Part model, mm, in its own coordinate system. A direction names the side the tool comes from. Coordinates: 2 decimals unless noted, no trailing zeros. Write each loop counter-clockwise with the first axis right and the second up, starting at its lowest first coordinate (ties: lowest second). Pieces come first, ordered by that corner, then holes. Notation, with made-up numbers: M 13,19.5 L 31,19.5 A22 ccw 31,30.5 Z; hole C 29,70.5 d3. An arc over 180 degrees is marked long. Use a Markdown table: item, result. Add a question column.
Q1. Slice it at B-B on y = 60.5. Write the cut outline in (x, z).
Q2. Tool access for faces 4 (the flat face through (-27.1, 42, 0)), 5 (the flat face through (25, 33, 0)), 6 (the flat face through (28, 57, -5)), 7 (the cylindrical face through (-28.53, 42.536, 7.325)), 8 (the flat face through (-28, 31, -15)): list every direction of +Z, -Z, +X, -X, +Y, -Y with a clear straight run to the whole face (end or side of a thin tool).
Q3. Pin check, flat tips, straight feed: pin 1 Ø1 at (x, z) = (5, -26) entering from -Y; pin 2 Ø5 at (x, z) = (9.5, 37.5) entering from -Y; pin 3 Ø5.5 at (x, y) = (28, 53) entering from -Z; pin 4 Ø4 at (x, z) = (-8.49, 8.49) entering from +Y. Stop position of each tip, or through.
Q4. Wall check: L1, parallel to Y at x = -27.5, z = -0.5; L2, parallel to X at y = 1.25, z = 0; L3, parallel to X at y = 30.5, z = 11. Give the ranges that are in metal, low to high. Write a range as from..to.
Q5. Mould opens along X. For faces 1 (the cylindrical face through (-24, 6, 0)), 2 (the cylindrical face through (-27, 5, -17)), 3 (the cylindrical face through (-32, 5, 0)) say: released by +X, released by -X, zero draft, split by the parting line, or undercut.
Q6. Slice it at A-A on y = 30. Write the cut outline in (x, z).
from build123d import *

# Parameters (mm, degrees)
SKETCH1_R           = 62.5
SKETCH1_R_2         = 1.3
SKETCH1_R_3         = 1.6
BOSS_EXTRUDE1_DEPTH = 4
FILLET3_R           = 2
SKETCH4_R           = 6.25
CUT_EXTRUDE3_DEPTH  = 2.1
SKETCH5_W           = 5
SKETCH5_H           = 30
BOSS_EXTRUDE2_DEPTH = 70
CUT_EXTRUDE4_START  = -5
CUT_EXTRUDE4_DEPTH  = 5
FILLET4_R           = 10
CUT_EXTRUDE5_START  = -5
CUT_EXTRUDE5_DEPTH  = 5
FILLET5_R           = 10
SKETCH13_R          = 11.6
CUT_EXTRUDE7_DEPTH  = 2.1
CUT_EXTRUDE8_REACH  = 133.949
SKETCH14_R          = 1.6
SKETCH14_R_2        = 1.5
CUT_EXTRUDE10_REACH = 114.75
SKETCH16_R          = 7.5
CUT_EXTRUDE11_REACH = 135.935
FILLET7_R           = 5


# Read off the part's stored shape, not the designer's step: Cut-Extrude4, Cut-Extrude5
with BuildPart() as part:
    # Sketch1 → Boss-Extrude1 (new body)
    with BuildSketch(Plane(origin=(0, 0, 0), x_dir=(1, 0, 0), z_dir=(0, 1, 0))):
        with Locations(Location((0, 0, 0), (0, 0, 270))):
            Circle(SKETCH1_R)
        with Locations(Location((-12, 0, 0), (0, 0, 270))):
            Circle(SKETCH1_R_2, mode=Mode.SUBTRACT)
        with Locations(Location((-8.485281374, 8.485281374, 0), (0, 0, 270))):
            Circle(SKETCH1_R_2, mode=Mode.SUBTRACT)
        with Locations(Location((0, 12, 0), (0, 0, 270))):
            Circle(SKETCH1_R_2, mode=Mode.SUBTRACT)
        with Locations(Location((8.485281374, 8.485281374, 0), (0, 0, 270))):
            Circle(SKETCH1_R_2, mode=Mode.SUBTRACT)
        with Locations(Location((12, 0, 0), (0, 0, 270))):
            Circle(SKETCH1_R_2, mode=Mode.SUBTRACT)
        with Locations(Location((8.485281374, -8.485281374, 0), (0, 0, 270))):
            Circle(SKETCH1_R_2, mode=Mode.SUBTRACT)
        with Locations(Location((0, -12, 0), (0, 0, 270))):
            Circle(SKETCH1_R_2, mode=Mode.SUBTRACT)
        with Locations(Location((-8.485281374, -8.485281374, 0), (0, 0, 270))):
            Circle(SKETCH1_R_2, mode=Mode.SUBTRACT)
        with Locations(Location((0, 0, 0), (0, 0, 270))):
            Circle(SKETCH1_R_3, mode=Mode.SUBTRACT)
    extrude(amount=BOSS_EXTRUDE1_DEPTH)

    # Fillet3
    fillet3_edges = [part.edges().sort_by_distance(p)[0] for p in [
        (0, 0, -62.5),
        (0, 4, -62.5),
    ]]
    fillet(fillet3_edges, radius=FILLET3_R - 0.0001)  # a hair under: the kernel refuses the full size

    # Sketch4 → Cut-Extrude3 (cut)
    with BuildSketch(Plane.XZ):
        with Locations(Location((0, 0, 0), (0, 0, 270))):
            Circle(SKETCH4_R)
    extrude(amount=-CUT_EXTRUDE3_DEPTH, mode=Mode.SUBTRACT)

    # Sketch5 → Boss-Extrude2 (add)
    with BuildSketch(Plane(origin=(0, 4, 0), x_dir=(1, 0, 0), z_dir=(0, 1, 0))):
        with Locations((-27.5, 0)):
            Rectangle(SKETCH5_W, SKETCH5_H)
        with Locations((27.5, 0)):
            Rectangle(SKETCH5_W, SKETCH5_H)
    extrude(amount=BOSS_EXTRUDE2_DEPTH)

    # Cut-Extrude4 outline → Cut-Extrude4 (cut)
    with BuildSketch(Plane(origin=(30, 0, 0), x_dir=(0, 0, -1), z_dir=(1, 0, 0)).offset(CUT_EXTRUDE4_START)):
        with BuildLine():
            Line((-15, 56), (-4.1208356, 71.831733384))
            ThreePointArc((-4.1208356, 71.831733384), (-2.328232471, 73.424854072), (4.9e-08, 74))
            Line((4.9e-08, 74), (-15, 74))
            Line((-15, 74), (-15, 56))
        make_face()
        with BuildLine():
            Line((15, 74), (4.9e-08, 74))
            ThreePointArc((4.9e-08, 74), (2.328232515, 73.424854049), (4.1208356, 71.831733384))
            Line((4.1208356, 71.831733384), (15, 56))
            Line((15, 56), (15, 74))
        make_face()
    extrude(amount=CUT_EXTRUDE4_DEPTH, mode=Mode.SUBTRACT)

    # Fillet4
    fillet4_edges = [part.edges().sort_by_distance(p)[0] for p in [
        (27.5, 56, 15),
        (27.5, 56, -15),
    ]]
    fillet(fillet4_edges, radius=FILLET4_R)

    # Cut-Extrude5 outline → Cut-Extrude5 (cut)
    with BuildSketch(Plane.ZY.offset(30).offset(CUT_EXTRUDE5_START)):
        with BuildLine():
            Line((-15, 56), (-4.1208356, 71.831733384))
            ThreePointArc((-4.1208356, 71.831733384), (-2.328232471, 73.424854072), (4.9e-08, 74))
            Line((4.9e-08, 74), (-15, 74))
            Line((-15, 74), (-15, 56))
        make_face()
        with BuildLine():
            Line((15, 74), (4.9e-08, 74))
            ThreePointArc((4.9e-08, 74), (2.328232515, 73.424854049), (4.1208356, 71.831733384))
            Line((4.1208356, 71.831733384), (15, 56))
            Line((15, 56), (15, 74))
        make_face()
    extrude(amount=CUT_EXTRUDE5_DEPTH, mode=Mode.SUBTRACT)

    # Fillet5
    fillet5_edges = [part.edges().sort_by_distance(p)[0] for p in [
        (-27.5, 56, -15),
        (-27.5, 56, 15),
    ]]
    fillet(fillet5_edges, radius=FILLET5_R)

    # Sketch13 → Cut-Extrude7 (cut)
    with BuildSketch(Plane(origin=(-25, 0, 0), x_dir=(0, 0, -1), z_dir=(1, 0, 0))):
        with Locations((0, 44)):
            Circle(SKETCH13_R)
    extrude(amount=-CUT_EXTRUDE7_DEPTH, mode=Mode.SUBTRACT)

    # Sketch14 → Cut-Extrude8 (cut, up to next)
    with BuildSketch(Plane(origin=(-27.1, 0, 0), x_dir=(0, 0, -1), z_dir=(1, 0, 0)), mode=Mode.PRIVATE) as cut_extrude8_sk1:
        with Locations((0, 44)):
            Circle(SKETCH14_R)
    cut_extrude8_tool1 = extrude(cut_extrude8_sk1.sketch, amount=-CUT_EXTRUDE8_REACH, mode=Mode.PRIVATE) & part.part
    # Sketch14 → Cut-Extrude8 (cut, up to next)
    with BuildSketch(Plane(origin=(-27.1, 0, 0), x_dir=(0, 0, -1), z_dir=(1, 0, 0)), mode=Mode.PRIVATE) as cut_extrude8_sk2:
        with Locations((0, 51)):
            Circle(SKETCH14_R_2)
    cut_extrude8_tool2 = extrude(cut_extrude8_sk2.sketch, amount=-CUT_EXTRUDE8_REACH, mode=Mode.PRIVATE) & part.part
    # Sketch14 → Cut-Extrude8 (cut, up to next)
    with BuildSketch(Plane(origin=(-27.1, 0, 0), x_dir=(0, 0, -1), z_dir=(1, 0, 0)), mode=Mode.PRIVATE) as cut_extrude8_sk3:
        with Locations((7, 44)):
            Circle(SKETCH14_R_2)
    cut_extrude8_tool3 = extrude(cut_extrude8_sk3.sketch, amount=-CUT_EXTRUDE8_REACH, mode=Mode.PRIVATE) & part.part
    # Sketch14 → Cut-Extrude8 (cut, up to next)
    with BuildSketch(Plane(origin=(-27.1, 0, 0), x_dir=(0, 0, -1), z_dir=(1, 0, 0)), mode=Mode.PRIVATE) as cut_extrude8_sk4:
        with Locations((0, 37)):
            Circle(SKETCH14_R_2)
    cut_extrude8_tool4 = extrude(cut_extrude8_sk4.sketch, amount=-CUT_EXTRUDE8_REACH, mode=Mode.PRIVATE) & part.part
    # Sketch14 → Cut-Extrude8 (cut, up to next)
    with BuildSketch(Plane(origin=(-27.1, 0, 0), x_dir=(0, 0, -1), z_dir=(1, 0, 0)), mode=Mode.PRIVATE) as cut_extrude8_sk5:
        with Locations((-7, 44)):
            Circle(SKETCH14_R_2)
    cut_extrude8_tool5 = extrude(cut_extrude8_sk5.sketch, amount=-CUT_EXTRUDE8_REACH, mode=Mode.PRIVATE) & part.part
    add(cut_extrude8_tool1.solids().sort_by_distance((-27.1, 44, 0))[0], mode=Mode.SUBTRACT)
    add(cut_extrude8_tool2.solids().sort_by_distance((-27.1, 51, 0))[0], mode=Mode.SUBTRACT)
    add(cut_extrude8_tool3.solids().sort_by_distance((-27.1, 44, -7))[0], mode=Mode.SUBTRACT)
    add(cut_extrude8_tool4.solids().sort_by_distance((-27.1, 37, 0))[0], mode=Mode.SUBTRACT)
    add(cut_extrude8_tool5.solids().sort_by_distance((-27.1, 44, 7))[0], mode=Mode.SUBTRACT)

    # Sketch16 → Cut-Extrude10 (cut, up to next)
    with BuildSketch(Plane(origin=(0, 4, 0), x_dir=(1, 0, 0), z_dir=(0, 1, 0)), mode=Mode.PRIVATE) as cut_extrude10_sk1:
        with Locations(Location((0, 30, 0), (0, 0, 270))):
            Circle(SKETCH16_R)
    cut_extrude10_tool1 = extrude(cut_extrude10_sk1.sketch, amount=-CUT_EXTRUDE10_REACH, mode=Mode.PRIVATE) & part.part
    add(cut_extrude10_tool1.solids().sort_by_distance((0, 4, -30))[0], mode=Mode.SUBTRACT)

    # Sketch18 → Cut-Extrude11 (cut, up to next)
    with BuildSketch(Plane(origin=(30, 0, 0), x_dir=(0, 0, -1), z_dir=(1, 0, 0)), mode=Mode.PRIVATE) as cut_extrude11_sk1:
        with BuildLine():
            Line((5, 74), (5, 44))
            ThreePointArc((5, 44), (0, 39), (-5, 44))
            Line((-5, 44), (-5, 74))
            ThreePointArc((-5, 74), (0, 79), (5, 74))
        make_face()
    cut_extrude11_tool1 = extrude(cut_extrude11_sk1.sketch, amount=-CUT_EXTRUDE11_REACH, mode=Mode.PRIVATE) & part.part
    add(cut_extrude11_tool1.solids().sort_by_distance((30, 59, 0))[0], mode=Mode.SUBTRACT)

    # Fillet7
    fillet7_edges = [part.edges().sort_by_distance(p)[0] for p in [
        (-25, 4, 0),
        (-27.5, 4, -15),
        (-30, 4, 0),
        (-27.5, 4, 15),
        (30, 4, 0),
        (27.5, 4, -15),
        (25, 4, 0),
        (27.5, 4, 15),
    ]]
    fillet(fillet7_edges, radius=FILLET7_R)


solid = part.part
Recorded:
| question | item | result |
|---|---|---|
| 1 | outline | M -30,-11.91 L -25,-11.91 L -25,11.91 L -30,11.91 Z; M 25,-11.91 L 30,-11.91 L 30,-5 L 25,-5 Z; M 25,5 L 30,5 L 30,11.91 L 25,11.91 Z |
| 2 | face 4 | none |
| 2 | face 5 | +Z, -Z, +Y |
| 2 | face 6 | +X, +Y |
| 2 | face 7 | -X |
| 2 | face 8 | -Z, +X, -X, +Y |
| 3 | pin 1 | through |
| 3 | pin 2 | y = 0 |
| 3 | pin 3 | z = -15 |
| 3 | pin 4 | y = 4 |
| 4 | L1 | 0..35.59, 38.41..42.48, 45.52..49.59, 52.41..73.97 |
| 4 | L2 | -62.35..-13.3, -10.7..-6.25, 6.25..10.7, 13.3..62.35 |
| 4 | L3 | -30..-25, 25..30 |
| 5 | face 1 | undercut |
| 5 | face 2 | zero draft |
| 5 | face 3 | released by -X |
| 6 | outline | M -30,-15 L -25,-15 L -25,15 L -30,15 Z; M 25,-15 L 30,-15 L 30,15 L 25,15 Z |
